Part model, mm, in its own coordinate system. A direction names the side the tool comes from. Round coordinates to 2 decimals unless told otherwise and drop trailing zeros. Loops run counter-clockwise (first coordinate to the right, second up) from the corner with the lowest first, then second, coordinate; pieces in that order, holes last.
(1) Probe probe 1 along X at (y, z) = (21.5, 4.95); probe 2 along Z at (x, y) = (-13, 14) (3 decimals); probe 3 along X at (y, z) = (7, -8). List the from-to ranges inside material, lowest first.
(2) Cut at C-C on y = 19. List the corners of the cut face in (x, z) (3 decimals), then the cut area to 3 significant figures.
(3) Cut at D-D on z = 4.95. List the corners of the cut face in (x, y), then the cut area to 3 significant figures.
(4) Flat gauge pins, fed straight in: pin 1 (11 mm diameter, centred on x = 0.5, z = -3.5, fed in from +Y); pin 2 (1.1 mm diameter, centred on x = -1.5, y = 30.5, fed in from +Z) (3 decimals); pin 3 (0.5 mm diameter, centred on x = 4, y = 30.5, fed in from -Z). Where does each tip first touch, or does it go through?
(5) Cut at A-A on z = -7. List the corners of the cut face in (x, y).
(6) Cut at B-B on x = -24.35. List the corners of the cut face in (y, z) (3 decimals), then the cut area to 3 significant figures.
(7) Tool access for faces 1 (the face through (-24, 18.1, -5)), 2 (the face through (-20.08, 21, 0)), 3 (the face through (-0.582, 30.593, -13.676)), 4 (the face through (0, 0, 0)), 5 (the face through (-24.39, 13.14, 8.99)): list every direction of +Z, -Z, +X, -X, +Y, -Y with a clear straight run to the whole face (end or side of a thin tool).
(8) Mould opens along X. For faces 6 (the face through (-28.58, 15, -4)), 7 (the face through (-24, 12, -2)), 8 (the face through (-23.423, 24.184, -4.744)) say: +X half, -X half, draft (parallel to the pull), parting line (faces both ways), or undercut.
from build123d import *

# Parameters (mm, degrees)
SKETCH1_W           = 57.16
SKETCH1_H           = 37.39
SKETCH1_W_2         = 40.16
SKETCH1_H_2         = 20.39
BOSS_EXTRUDE1_DEPTH = 2
SKETCH2_W           = 57.16
SKETCH2_H           = 37.39
SKETCH2_W_2         = 40.16
SKETCH2_H_2         = 20.39
BOSS_EXTRUDE2_DEPTH = 28.1
SKETCH3_W           = 48.66
SKETCH3_H           = 8.5
CUT_EXTRUDE1_DEPTH  = 28.1
CUT_EXTRUDE2_REACH  = 62.194
SKETCH5_W           = 20.39
SKETCH5_H           = 10
FILLET1_R           = 4
SKETCH6_R           = 0.95
CUT_EXTRUDE3_DEPTH  = 12
SKETCH7_W           = 0.569871794
SKETCH7_H           = 3.175
BOSS_EXTRUDE3_DEPTH = 1


with BuildPart() as part:
    # Sketch1 → Boss-Extrude1 (new body)
    # profile 1 of 2: a face of its own
    with BuildSketch(Plane(origin=(0, 0, 0), x_dir=(1, 0, 0), z_dir=(0, 1, 0))):
        Rectangle(SKETCH1_W, SKETCH1_H)
        Rectangle(SKETCH1_W_2, SKETCH1_H_2, mode=Mode.SUBTRACT)
    # profile 2 of 2: a face of its own
    with BuildSketch(Plane(origin=(0, 0, 0), x_dir=(1, 0, 0), z_dir=(0, 1, 0))):
        Rectangle(SKETCH1_W_2, SKETCH1_H_2)
    extrude(amount=BOSS_EXTRUDE1_DEPTH)

    # Sketch2 → Boss-Extrude2 (add)
    with BuildSketch(Plane(origin=(0, 2, 0), x_dir=(1, 0, 0), z_dir=(0, 1, 0))):
        Rectangle(SKETCH2_W, SKETCH2_H)
        Rectangle(SKETCH2_W_2, SKETCH2_H_2, mode=Mode.SUBTRACT)
    extrude(amount=BOSS_EXTRUDE2_DEPTH)

    # Sketch3 → Cut-Extrude1 (cut)
    with BuildSketch(Plane(origin=(0, 30.1, 0), x_dir=(1, 0, 0), z_dir=(0, 1, 0))):
        with Locations((-4.25, -14.445)):
            Rectangle(SKETCH3_W, SKETCH3_H)
    extrude(amount=-CUT_EXTRUDE1_DEPTH, mode=Mode.SUBTRACT)

    # Sketch5 → Cut-Extrude2 (cut, up to next)
    with BuildSketch(Plane(origin=(-20.08, 0, 0), x_dir=(0, 0, -1), z_dir=(1, 0, 0)), mode=Mode.PRIVATE) as cut_extrude2_sk1:
        with Locations((0, 7)):
            Rectangle(SKETCH5_W, SKETCH5_H)
    cut_extrude2_tool1 = extrude(cut_extrude2_sk1.sketch, amount=-CUT_EXTRUDE2_REACH, mode=Mode.PRIVATE) & part.part
    add(cut_extrude2_tool1.solids().sort_by_distance((-20.08, 7, 0))[0], mode=Mode.SUBTRACT)

    # Fillet1
    fillet1_edges = [part.edges().sort_by_distance(p)[0] for p in [
        (-24.33, 12, 10.195),
    ]]
    fillet(fillet1_edges, radius=FILLET1_R)

    # Sketch6 → Cut-Extrude3 (cut)
    with BuildSketch(Plane(origin=(0, 30.1, 0), x_dir=(1, 0, 0), z_dir=(0, 1, 0))):
        with Locations(Location((-24.35, -4.95, 0), (0, 0, 270))):
            Circle(SKETCH6_R)
        with Locations(Location((-24.35, 4.95, 0), (0, 0, 90))):
            Circle(SKETCH6_R)
        with Locations(Location((24.35, 4.95, 0), (0, 0, 270))):
            Circle(SKETCH6_R)
        with Locations(Location((24.35, -4.95, 0), (0, 0, 90))):
            Circle(SKETCH6_R)
    extrude(amount=-CUT_EXTRUDE3_DEPTH, mode=Mode.SUBTRACT)

    # Sketch7 → Boss-Extrude3 (add)
    # profile 1 of 4: a face of its own
    with BuildSketch(Plane(origin=(0, 30.1, 0), x_dir=(1, 0, 0), z_dir=(0, 1, 0))):
        with BuildLine():
            Line((-5.16235185, 15.241554144), (-4.526334221, 15.241554144))
            add(Edge.make_bspline(
                [(-4.526334221, 15.241554144), (-4.484777655, 15.241368128), (-4.404606327, 15.241009264), (-4.288992676, 15.236657561), (-4.182333422, 15.228859045), (-4.08465307, 15.219221313), (-3.995991784, 15.205709587), (-3.916238533, 15.190219451), (-3.845376767, 15.171347958), (-3.782607413, 15.148947756), (-3.726273946, 15.122538794), (-3.672964317, 15.094411364), (-3.623883329, 15.060842269), (-3.576553717, 15.025449442), (-3.533681396, 14.984851821), (-3.492591735, 14.941751237), (-3.455024992, 14.894438355), (-3.420807097, 14.843485885), (-3.389766194, 14.789835212), (-3.362646785, 14.733390423), (-3.340649039, 14.6740622), (-3.322195665, 14.612234331), (-3.307373735, 14.547909509), (-3.297507787, 14.48069213), (-3.290806339, 14.411051534), (-3.290215029, 14.363654099), (-3.289915952, 14.339681147)],
                knots=[0, 0, 0, 0, 1.698747864, 3.27724071, 4.728299578, 6.070144658, 7.288476769, 8.393259625, 9.389771311, 10.283485332, 11.113357557, 11.931608583, 12.74405601, 13.541433047, 14.344816069, 15.154114104, 15.974336324, 16.810834471, 17.661136416, 18.50621059, 19.367396281, 20.244825668, 21.142564693, 22.063065223, 23.020325768, 24, 24, 24, 24], degree=3))
            add(Edge.make_bspline(
                [(-3.289915952, 14.339681147), (-3.290348678, 14.313160441), (-3.291199038, 14.261043994), (-3.299535306, 14.184647677), (-3.313776285, 14.111810705), (-3.332388499, 14.041918832), (-3.358341909, 13.976121933), (-3.38799246, 13.912850075), (-3.424472043, 13.853877205), (-3.466155799, 13.798465646), (-3.511679216, 13.746164873), (-3.562123017, 13.698484974), (-3.616525724, 13.655100917), (-3.674572416, 13.615558031), (-3.73648102, 13.579936086), (-3.802206865, 13.547901518), (-3.872198765, 13.520478893), (-3.920939018, 13.506137082), (-3.945650127, 13.498865843)],
                knots=[0, 0, 0, 0, 1.102006807, 2.165578795, 3.188629044, 4.184801286, 5.166646146, 6.124351954, 7.085497154, 8.042432466, 9.003981491, 9.963833307, 10.922997304, 11.89326795, 12.880200226, 13.889073926, 14.929769137, 16, 16, 16, 16], degree=3))
            add(Edge.make_bspline(
                [(-3.945650127, 13.498865843), (-3.961926284, 13.494816308), (-3.997185683, 13.486043713), (-4.055530303, 13.477137327), (-4.122766351, 13.468948452), (-4.199111247, 13.461911106), (-4.284609004, 13.45712735), (-4.379176838, 13.45339145), (-4.482857606, 13.450675064), (-4.554953112, 13.450578675), (-4.592480055, 13.450528503)],
                knots=[0, 0, 0, 0, 0.618981996, 1.340914327, 2.176866532, 3.120127938, 4.170906482, 5.338178032, 6.614476169, 8, 8, 8, 8], degree=3))
            Line((-4.592480055, 13.450528503), (-4.592480055, 12.066554144))
            Line((-4.592480055, 12.066554144), (-5.16235185, 12.066554144))
            Line((-5.16235185, 12.066554144), (-5.16235185, 15.241554144))
        make_face()
        with BuildLine():
            Line((-4.592480055, 14.020400298), (-4.390862467, 14.020400298))
            add(Edge.make_bspline(
                [(-4.390862467, 14.020400298), (-4.354174963, 14.020632925), (-4.286669412, 14.021060962), (-4.194480668, 14.027250635), (-4.12039602, 14.036703515), (-4.061867772, 14.050261131), (-4.015654177, 14.070836608), (-3.975797844, 14.094638561), (-3.94161205, 14.124735477), (-3.912012184, 14.159126353), (-3.888347983, 14.198643193), (-3.871938093, 14.242642543), (-3.86127855, 14.290199928), (-3.860294043, 14.323296721), (-3.859787747, 14.340317165)],
                knots=[0, 0, 0, 0, 1.8619151, 3.425951444, 4.686033666, 5.651700536, 6.461346321, 7.243864085, 7.999046032, 8.762387399, 9.539336099, 10.322741239, 11.137448474, 12, 12, 12, 12], degree=3))
            add(Edge.make_bspline(
                [(-3.859787747, 14.340317165), (-3.860288835, 14.355187705), (-3.861261065, 14.384040128), (-3.868403335, 14.425681332), (-3.879786058, 14.464499524), (-3.896279186, 14.5000893), (-3.917600896, 14.532390187), (-3.943596375, 14.56138946), (-3.973932049, 14.587708164), (-3.997352964, 14.601639056), (-4.00925189, 14.608716604)],
                knots=[0, 0, 0, 0, 1.102301479, 2.1387299, 3.123554645, 4.094223062, 5.036071848, 5.982632524, 6.975082478, 8, 8, 8, 8], degree=3))
            add(Edge.make_bspline(
                [(-4.00925189, 14.608716604), (-4.019330967, 14.613813882), (-4.040670438, 14.624605865), (-4.077013627, 14.637152333), (-4.118953111, 14.647736662), (-4.166772031, 14.656521552), (-4.220279622, 14.66333954), (-4.279466337, 14.668553594), (-4.344419277, 14.670650369), (-4.38959016, 14.671328868), (-4.413123084, 14.671682349)],
                knots=[0, 0, 0, 0, 0.656809284, 1.390599849, 2.23162475, 3.173112763, 4.218524733, 5.370385145, 6.63003504, 8, 8, 8, 8], degree=3))
            Line((-4.413123084, 14.671682349), (-4.592480055, 14.671682349))
            Line((-4.592480055, 14.671682349), (-4.592480055, 14.020400298))
        make_face(mode=Mode.SUBTRACT)
    # profile 2 of 4: a face of its own
    with BuildSketch(Plane(origin=(0, 30.1, 0), x_dir=(1, 0, 0), z_dir=(0, 1, 0))):
        Polygon((-1.743757098, 15.241554144), (-1.213954414, 15.241554144), (0.068257125, 12.066554144), (-0.540411746, 12.066554144), (-0.787186585, 12.717836195), (-2.169252891, 12.717836195), (-2.416663749, 12.066554144), (-3.025332619, 12.066554144), align=None)
        Polygon((-1.478537747, 14.38992654), (-1.953006898, 13.28770799), (-1.003432579, 13.28770799), align=None, mode=Mode.SUBTRACT)
    # profile 3 of 4: a face of its own
    with BuildSketch(Plane(origin=(0, 30.1, 0), x_dir=(1, 0, 0), z_dir=(0, 1, 0))):
        with Locations((0.73989174, 13.654054144)):
            Rectangle(SKETCH7_W, SKETCH7_H)
    # profile 4 of 4: a face of its own
    with BuildSketch(Plane(origin=(0, 30.1, 0), x_dir=(1, 0, 0), z_dir=(0, 1, 0))):
        Polygon((1.757519945, 15.241554144), (2.270786171, 15.241554144), (3.711366099, 13.152236235), (3.711366099, 15.241554144), (4.281237894, 15.241554144), (4.281237894, 12.066554144), (3.764155562, 12.066554144), (2.32739174, 14.149511876), (2.32739174, 12.066554144), (1.757519945, 12.066554144), align=None)
    extrude(amount=BOSS_EXTRUDE3_DEPTH)


solid = part.part
Final values:
1. probe 1: x = -28.58 to -25.3, -23.4 to -20.08, 20.08 to 23.4, 25.3 to 28.58
1. probe 2: z = -18.695 to -10.195
1. probe 3: x = 20.08 to 28.58
2. outline: (-28.58, -18.695) - (28.58, -18.695) - (28.58, 18.695) - (20.08, 18.695) - (20.08, -10.195) - (-20.08, -10.195) - (-20.08, 10.195) - (-28.58, 10.195) - close; hole circle Ø1.9 at (-24.35, -4.95); hole circle Ø1.9 at (-24.35, 4.95); hole circle Ø1.9 at (24.35, -4.95); hole circle Ø1.9 at (24.35, 4.95)
2. area: 893 mm2
3. outline: (-28.58, 0) - (28.58, 0) - (28.58, 30.1) - (25.3, 30.1) - (25.3, 18.1) - (23.4, 18.1) - (23.4, 30.1) - (20.08, 30.1) - (20.08, 2) - (-28.58, 2) - close; (-28.58, 12) - (-20.08, 12) - (-20.08, 30.1) - (-23.4, 30.1) - (-23.4, 18.1) - (-25.3, 18.1) - (-25.3, 30.1) - (-28.58, 30.1) - close
3. area: 461 mm2
4. pin 1: stops at y = 2
4. pin 2: stops at z = -10.195
4. pin 3: stops at z = -15.24
5. outline: (-28.58, 0) - (28.58, 0) - (28.58, 30.1) - (20.08, 30.1) - (20.08, 2) - (-28.58, 2) - close; (-28.58, 12) - (-20.08, 12) - (-20.08, 30.1) - (-28.58, 30.1) - close
6. outline: (0, -18.695) - (30.1, -18.695) - (30.1, -5.9) - (18.1, -5.9) - (18.1, -4) - (30.1, -4) - (30.1, 4) - (18.1, 4) - (18.1, 5.9) - (30.1, 5.9) - (30.1, 10.195) - (16, 10.195) arc R4 ccw to (12, 6.195) - (12, -10.195) - (2, -10.195) - (2, 18.695) - (0, 18.695) - close
6. area: 634 mm2
7. face 1: +Y
7. face 2: +Z, +Y
7. face 3: -Z, +Y
7. face 4: +Z, -Z, +X, -X, -Y
7. face 5: +Z, -X
8. face 6: -X half
8. face 7: draft
8. face 8: undercut
